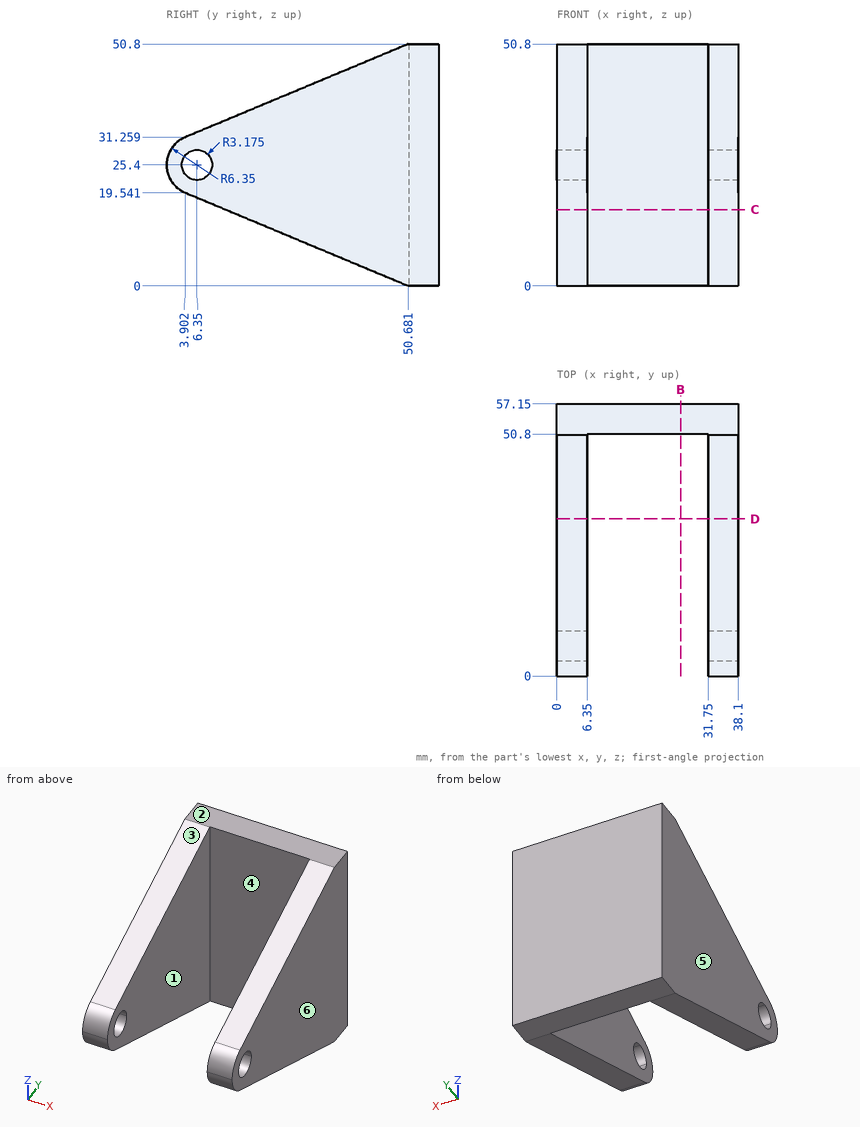
Study the drawing (mm; zero at the part's minimum x, y, z) and answer. A direction names the side the tool comes from. Coordinates: 2 decimals unless noted, no trailing zeros. Loops run counter-clockwise (first coordinate to the right, second up) from the corner with the lowest first, then second, coordinate; pieces in that order, holes last. Notation, with made-up numbers: M 27,28.25 L 37,28.25 A22 ccw 37,47.25 Z; hole C 60,-31.75 d8. An arc over 180 degrees is marked long. Answer in a Markdown table with one row per item.
1) Find section B-B (x = 26). Determine the outline of the cut face in (y, z).
Answers below:
| item | result |
|---|---|
| outline | M 50.8,0 L 57.15,0 L 57.15,50.8 L 50.8,50.8 Z |
2) Determine the mould class of the marked faces 3, 4, 5 and 6 for opening direction X: released by +X, released by -X, zero draft, split by the parting line, or undercut.
Answers below:
| item | result |
|---|---|
| face 3 | zero draft |
| face 4 | undercut |
| face 5 | released by -X |
| face 6 | released by +X |
3) Which of the six approach directions +Z, -Z, +X, -X, +Y, -Y give full straight-line access (tool end or side, diameter ignored) to the marked faces 1 and 2?
Answers below:
| item | result |
|---|---|
| face 1 | +Z, -Z, -Y |
| face 2 | +Z, +X, -X, +Y, -Y |
4) Find the intervals of material crossed by probe 1 along X at (y, z) = (7, 29); probe 2 along Y at (x, z) = (17.5, 3.5); probe 3 along Z at (x, y) = (5, 5) (1 decimal), in increasing order.
Answers below:
| item | result |
|---|---|
| probe 1 | 0 to 6.35, 31.75 to 38.1 |
| probe 2 | 50.8 to 57.15 |
| probe 3 | 19.1 to 22.5, 28.3 to 31.7 |
5) Given pin 1 (7.5 mm diameter, centred on x = 15, z = 37.5, fed in from -Y); pin 2 (8 mm diameter, centred on x = 11.5, y = 43, fed in from -Z), each flat-ended and moving along its own axis, determine where each tip first touches the part or whether it passes through.
Answers below:
| item | result |
|---|---|
| pin 1 | y = 50.8 |
| pin 2 | through |
6) Find section C-C (z = 16). Determine the outline of the cut face in (x, y), then the cut area to 3 significant figures.
Answers below:
| item | result |
|---|---|
| outline | M 0,12.38 L 6.35,12.38 L 6.35,50.8 L 31.75,50.8 L 31.75,12.38 L 38.1,12.38 L 38.1,57.15 L 0,57.15 Z |
| area | 730 mm^2 |
7) Find section D-D (y = 33). Determine the outline of the cut face in (x, z).
Answers below:
| item | result |
|---|---|
| outline | M 0,7.39 L 6.35,7.39 L 6.35,43.41 L 0,43.41 Z; M 31.75,7.39 L 38.1,7.39 L 38.1,43.41 L 31.75,43.41 Z |
